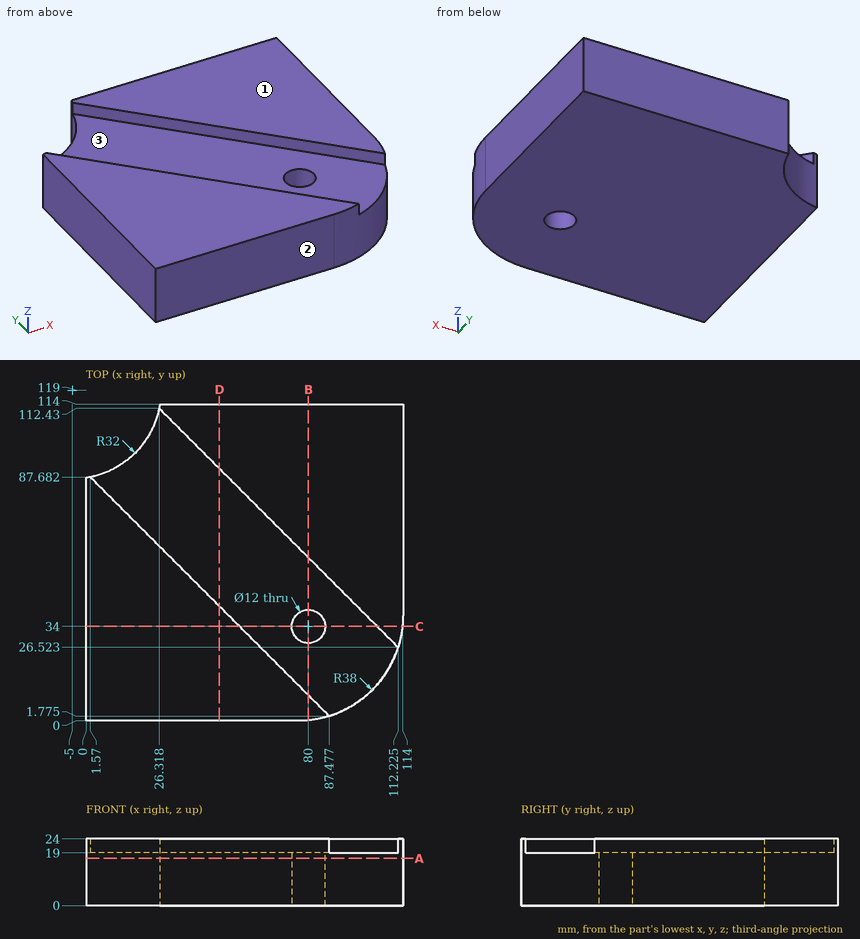
Job drawing, mm, ordinate dimensions from the low corner. One solid piece. Coordinates: 2 decimals unless noted, no trailing zeros. Order: outer loops, then holes, each group sorted by start corner. A loop starts at its lowest first (then second) coordinate and runs counter-clockwise, first axis right, second up. Notation, with made-up numbers: (52.5, 0.5) - (107.5, 0.5) arc R23 cw to (107.5, 16.5) - close; hole circle Ø5 at (89.25, -17.5). An arc over 180 degrees is marked (long way). Return JSON: item names as keys, results as strings. Group by question number.
1) Mould opens along Y. For the marked faces 1, 2 and 3 say: released by +Y, released by -Y, zero draft, split by the parting line, or undercut.
2) Probe line 1 (X direction, y = 34, z = 11.25); line 2 (Y direction, x = 40.5, z = 22.75); line 3 (X direction, y = 63, z = 21.5). List the from-to ranges inside material, lowest first. Write a range as from..to.
3) Saw through at C-C, the plane y = 34. Write the cut outline in (x, z), plus the area to 3 significant figures.
4) Saw through at B-B, the plane x = 80. Write the cut outline in (y, z), plus the area to 3 significant figures.
5) Saw through at A-A, the plane z = 17. Write the cut outline in (x, y).
6) Saw through at D-D, the plane x = 48. Write the cut outline in (y, z).
7) Flat gauge pins, fed straight in: P1, Ø14, axis at x = 80, y = 34, coming from the -Z side; P2, Ø2, axis at y = 99, z = 5.5, coming from the -X side (1 decimal). Where does each tip first touch, or does it go through?
Values found:
{
 "1": {"face 1": "zero draft", "face 2": "released by -Y", "face 3": "undercut"},
 "2": {"line 1": "x = 0..74, 86..113.79", "line 2": "y = 0..48.75, 98.25..114", "line 3": "x = 0..26.25, 75.75..114"},
 "3": {"outline": "(0, 0) - (74, 0) - (74, 19) - (55.25, 19) - (55.25, 24) - (0, 24) - close; (86, 0) - (113.79, 0) - (113.79, 24) - (104.75, 24) - (104.75, 19) - (86, 19) - close", "area": "2,260 mm²"},
 "4": {"outline": "(0.21, 0) - (28, 0) - (28, 19) - (9.25, 19) - (9.25, 24) - (0.21, 24) - close; (40, 0) - (114, 0) - (114, 24) - (58.75, 24) - (58.75, 19) - (40, 19) - close", "area": "2,260 mm²"},
 "5": {"outline": "(0, 0) - (76, 0) arc R38 ccw to (114, 38) - (114, 114) - (26.61, 114) arc R32 cw to (0, 87.39) - close; hole circle Ø12 at (80, 34)"},
 "6": {"outline": "(0, 0) - (114, 0) - (114, 24) - (90.75, 24) - (90.75, 19) - (41.25, 19) - (41.25, 24) - (0, 24) - close"},
 "7": {"P1": "stops at z = 0", "P2": "stops at x = 19.1"}
}
